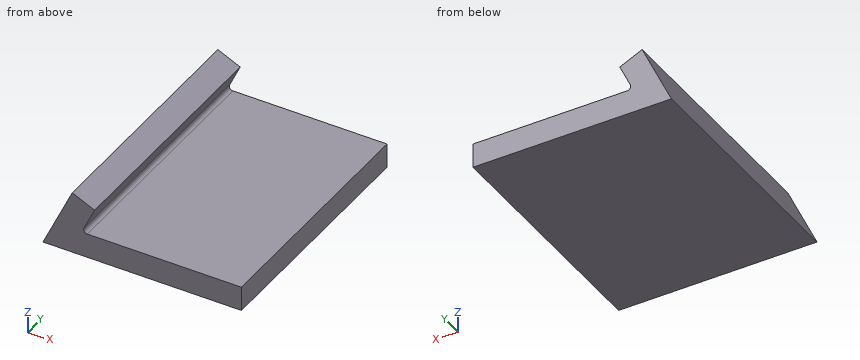
from build123d import *

# Parameters (mm, degrees)
F1_DEPTH = 20


with BuildPart() as f1:
    # F0 (on Front) → F1 (new body)
    with BuildSketch(Plane.XZ):
        with BuildLine():
            Line((2.383301, 5.111006), (0, 0))
            Line((0, 0), (16.139371, 0))
            Line((16.139371, 0), (16.139371, 2))
            Line((16.139371, 2), (3.601872, 2))
            ThreePointArc((3.601872, 2), (3.35337, 2.136333), (3.334832, 2.419168))
            Line((3.334832, 2.419168), (4.195917, 4.265769))
            Line((4.195917, 4.265769), (2.383301, 5.111006))
        make_face()
    extrude(amount=F1_DEPTH)


solid = f1.part
For this review, take the finished solid that the model builds, in its own axes (mm). Round coordinates to 2 decimals unless told otherwise and drop trailing zeros. Order: outer loops, then holes, each group sorted by start corner. A loop starts at its lowest first (then second) coordinate and runs counter-clockwise, first axis right, second up. Notation, with made-up numbers: M 8,29.5 L 52,29.5 A23 cw 52,37.5 Z; hole C 23.5,-15.75 d10. An arc over 180 degrees is marked long. Use a Markdown table: item, result. Add a question column.
Item 1: To check wall thickness, follow line 1 along Z through (x, y) = (8.75, -8); line 2 along Z through (x, y) = (3.75, -7.75); line 3 along Z through (x, y) = (3.5, -11.25). State the ranges of each line that lie inside material, in increasing order.
Item 2: Add section B-B, the plane x = 8. Give the boundary of the cut face in (y, z), then the cut area to 3 significant figures.
Item 3: Add section A-A, the plane y = -5.5. Give the boundary of the cut face in (x, z).
Item 4: Insertion check: pin 1 (1.5 mm diameter, centred on x = 13.5, y = -10.5, fed in from +Z). The pin has a flat end and moves straight along its axis. Give the tip position at first contact, or say it passes through.
Item 5: Add section C-C, the plane z = 2.75. Give the boundary of the cut face in (x, y).
Geometry results:
| question | item | result |
|---|---|---|
| 1 | line 1 | z = 0 to 2 |
| 1 | line 2 | z = 0 to 2, 3.31 to 4.47 |
| 1 | line 3 | z = 0 to 2.02, 2.77 to 4.59 |
| 2 | outline | M -20,0 L 0,0 L 0,2 L -20,2 Z |
| 2 | area | 40.0 mm² |
| 3 | outline | M 0,0 L 16.14,0 L 16.14,2 L 3.6,2 A0.29 cw 3.33,2.42 L 4.2,4.27 L 2.38,5.11 Z |
| 4 | pin 1 | stops at z = 2 |
| 5 | outline | M 1.28,-20 L 3.49,-20 L 3.49,0 L 1.28,0 Z |
